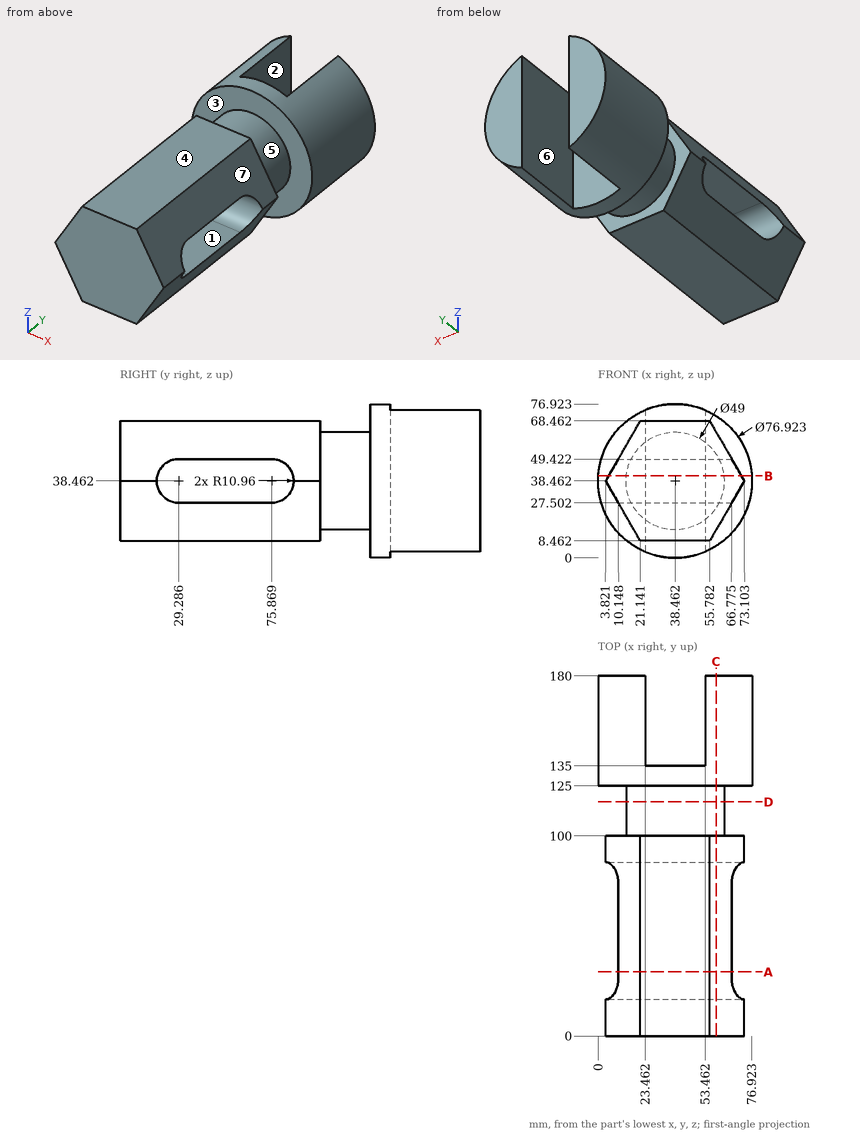
Part print with two shaded views. Sizes in mm from the minimum x, y, z corner. A direction names the side the tool comes from. Coordinates: 2 decimals unless noted, no trailing zeros. Write each loop counter-clockwise with the first axis right and the second up, starting at its lowest first coordinate (ties: lowest second). Pieces come first, ordered by that corner, then holes. Notation, with made-up numbers: (79, 79.25) - (98, 79.25) arc R13 cw to (98, 97.25) - close; hole circle Ø7 at (5, 38.5). An arc over 180 degrees is marked (long way). Put each result on its own line as item: value.
1. Band-saw the part on A-A (y = 32). Write the cut outline in (x, z) (1 decimal).
Final values:
outline: (10.1, 27.5) - (21.1, 8.5) - (55.8, 8.5) - (66.8, 27.5) - close; (10.1, 49.4) - (66.8, 49.4) - (55.8, 68.5) - (21.1, 68.5) - close
2. 3-axis set-ups, long thin cutter, end or side, ignore diameter. For the marked faces 1, 2, 3 and 4: which of +Z, -Z, +X, -X, +Y, -Y reach the whole face in a straight line?
Final values:
face 1: +X, -X
face 2: +Z, -Z, +Y
face 3: none
face 4: +Z, +X, -X, -Y
3. Band-saw the part on D-D (y = 117). Write the cut outline in (x, z).
Final values:
outline: circle Ø49 at (38.46, 38.46)
4. Probe line 1 along Z through (x, y) = (29, 98.5); line 2 along Y through (x, z) = (19, 5.5); line 3 along Y through (x, z) = (49, 67.5). List the from-to ranges inside material, lowest first. Write a range as [from, to].
Final values:
line 1: z = [8.46, 68.46]
line 2: y = [125, 180]
line 3: y = [0, 100], [125, 135]
5. Band-saw the part on B-B (z = 41). Write the cut outline in (x, y).
Final values:
outline: (0.08, 125) - (14.09, 125) - (14.09, 100) - (5.29, 100) - (5.29, 86.53) - (71.64, 86.53) - (71.64, 100) - (62.83, 100) - (62.83, 125) - (76.84, 125) - (76.84, 180) - (53.46, 180) - (53.46, 135) - (23.46, 135) - (23.46, 180) - (0.08, 180) - close; (5.29, 0) - (71.64, 0) - (71.64, 18.62) - (5.29, 18.62) - close
6. Two-plate mould, pull along X, no slides. Class the marked faces 5, 6 and 7: +X half, -X half, draft (parallel to the pull), parting line (faces both ways), or undercut.
Final values:
face 5: parting line
face 6: undercut
face 7: +X half
7. Flat gauge pins, fed straight in: pin 1 Ø1.5 at (x, y) = (24.5, 101.5) entering from -Z; pin 2 Ø12 at (x, y) = (45, 34) entering from -Z; pin 3 Ø1.5 at (x, z) = (24.5, 68.5) entering from +Y. Where does each tip first touch, or does it go through?
Final values:
pin 1: stops at z = 17.83
pin 2: stops at z = 8.46
pin 3: stops at y = 135
8. Band-saw the part on C-C (x = 59). Write the cut outline in (y, z) (1 decimal), then the cut area to 3 significant figures.
Final values:
outline: (0, 14) - (100, 14) - (100, 25.1) - (125, 25.1) - (125, 5.9) - (180, 5.9) - (180, 71) - (125, 71) - (125, 51.8) - (100, 51.8) - (100, 62.9) - (0, 62.9) - close; hole (29.3, 27.5) - (75.9, 27.5) arc R11 ccw to (75.9, 49.4) - (29.3, 49.4) arc R11 ccw to start
area: 7,730 mm²
